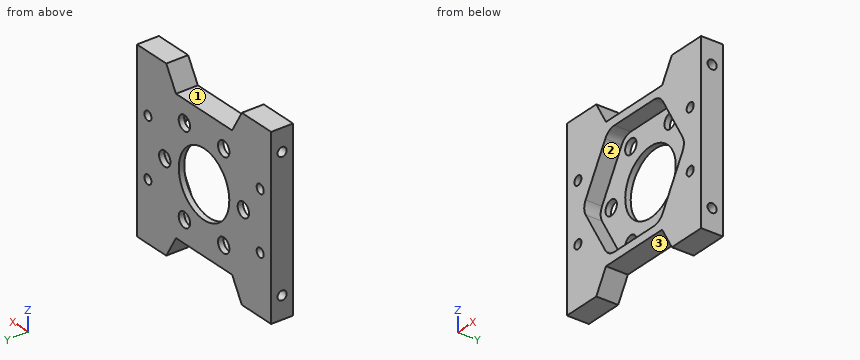
```python
from build123d import *

# Parameters (mm, degrees)
SKETCH_1_R          = 35
SKETCH_1_R_2        = 2.025
SKETCH_1_R_3        = 9
SKETCH_1_R_4        = 1.25
EXTRUDE_1_DEPTH     = 3
CUT_EXTRUDE_1_REACH = 51.86
SKETCH_2_R          = 35
SKETCH_2_W          = 47.8
SKETCH_2_H          = 48.2
SKETCH_3_R          = 1.25
CUT_EXTRUDE_2_DEPTH = 8
SKETCH_5_R          = 9
SKETCH_5_R_2        = 3.75
SKETCH_5_R_3        = 2.025
CUT_EXTRUDE_4_DEPTH = 4.5
CUT_EXTRUDE_6_DEPTH = 35.467666007


with BuildPart() as part:
    # 草图1 → 凸台-拉伸1 (new, symmetric)
    with BuildSketch(Plane(origin=(0, 0, 0), x_dir=(1, 0, 0), z_dir=(0, 1, 0))):
        with Locations(Location((0, 0, 0), (0, 0, 270))):
            Circle(SKETCH_1_R)
        with Locations(Location((14, 0, 0), (0, 0, 270))):
            Circle(SKETCH_1_R_2, mode=Mode.SUBTRACT)
        with Locations(Location((7, -12.124355653, 0), (0, 0, 270))):
            Circle(SKETCH_1_R_2, mode=Mode.SUBTRACT)
        with Locations(Location((-7, -12.124355653, 0), (0, 0, 270))):
            Circle(SKETCH_1_R_2, mode=Mode.SUBTRACT)
        with Locations(Location((-14, 0, 0), (0, 0, 270))):
            Circle(SKETCH_1_R_2, mode=Mode.SUBTRACT)
        with Locations(Location((-7, 12.124355653, 0), (0, 0, 270))):
            Circle(SKETCH_1_R_2, mode=Mode.SUBTRACT)
        with Locations(Location((7, 12.124355653, 0), (0, 0, 270))):
            Circle(SKETCH_1_R_2, mode=Mode.SUBTRACT)
        with Locations(Location((0, 0, 0), (0, 0, 270))):
            Circle(SKETCH_1_R_3, mode=Mode.SUBTRACT)
        with Locations(Location((-20, 8, 0), (0, 0, 270))):
            Circle(SKETCH_1_R_4, mode=Mode.SUBTRACT)
        with Locations(Location((-20, -8, 0), (0, 0, 90))):
            Circle(SKETCH_1_R_4, mode=Mode.SUBTRACT)
        with Locations(Location((20, -8, 0), (0, 0, 270))):
            Circle(SKETCH_1_R_4, mode=Mode.SUBTRACT)
        with Locations(Location((20, 8, 0), (0, 0, 90))):
            Circle(SKETCH_1_R_4, mode=Mode.SUBTRACT)
    extrude(amount=EXTRUDE_1_DEPTH, both=True)

    # 草图2 → 切除-拉伸1 (cut, up to next)
    with BuildSketch(Plane(origin=(0, 3, 0), x_dir=(1, 0, 0), z_dir=(0, 1, 0)), mode=Mode.PRIVATE) as cut_extrude_1_sk1:
        Circle(SKETCH_2_R)
        Rectangle(SKETCH_2_W, SKETCH_2_H, mode=Mode.SUBTRACT)
    cut_extrude_1_tool1 = extrude(cut_extrude_1_sk1.sketch, amount=-CUT_EXTRUDE_1_REACH, mode=Mode.PRIVATE) & part.part
    add(cut_extrude_1_tool1.solids().sort_by_distance((-34.010051, 3, 0))[0], mode=Mode.SUBTRACT)

    # 草图3 → 切除-拉伸2 (cut)
    with BuildSketch(Plane.ZY.offset(23.9)):
        with Locations((18, 0)):
            Circle(SKETCH_3_R)
        with Locations(Location((-18, 0, 0), (0, 0, 180))):
            Circle(SKETCH_3_R)
    cut_extrude_2 = extrude(amount=-CUT_EXTRUDE_2_DEPTH, mode=Mode.SUBTRACT)

    # 草图5 → 切除-拉伸4 (cut)
    # profile 1 of 7: a face of its own
    with BuildSketch(Plane.XZ.offset(3)):
        with BuildLine():
            Line((7, 15.874355653), (-7, 15.874355653))
            ThreePointArc((-7, 15.874355653), (-4.348349571, 14.776006082), (-3.25, 12.124355653))
            ThreePointArc((-3.25, 12.124355653), (-7.970571419, 8.502133804), (-10.247595264, 13.999355653))
            Line((-10.247595264, 13.999355653), (-17.247595264, 1.875))
            ThreePointArc((-17.247595264, 1.875), (-13.029428581, 3.622221849), (-10.25, 0))
            ThreePointArc((-10.25, 0), (-13.029428581, -3.622221849), (-17.247595264, -1.875))
            Line((-17.247595264, -1.875), (-10.247595264, -13.999355653))
            ThreePointArc((-10.247595264, -13.999355653), (-7.970571419, -8.502133804), (-3.25, -12.124355653))
            ThreePointArc((-3.25, -12.124355653), (-4.348349571, -14.776006082), (-7, -15.874355653))
            Line((-7, -15.874355653), (7, -15.874355653))
            ThreePointArc((7, -15.874355653), (4.348349571, -9.472705224), (10.75, -12.124355653))
            ThreePointArc((10.75, -12.124355653), (10.622221849, -13.094927072), (10.247595264, -13.999355653))
            Line((10.247595264, -13.999355653), (17.247595264, -1.875))
            ThreePointArc((17.247595264, -1.875), (10.25, 0), (17.247595264, 1.875))
            Line((17.247595264, 1.875), (10.247595264, 13.999355653))
            ThreePointArc((10.247595264, 13.999355653), (10.622221849, 13.094927072), (10.75, 12.124355653))
            ThreePointArc((10.75, 12.124355653), (4.348349571, 9.472705224), (7, 15.874355653))
        make_face()
        with Locations(Location((0, 0, 0), (0, 0, 270))):
            Circle(SKETCH_5_R, mode=Mode.SUBTRACT)
    # profile 2 of 7: a face of its own
    with BuildSketch(Plane.XZ.offset(3)):
        with Locations((-14, 0)):
            Circle(SKETCH_5_R_2)
        with Locations(Location((-14, 0, 0), (0, 0, 270))):
            Circle(SKETCH_5_R_3, mode=Mode.SUBTRACT)
    # profile 3 of 7: a face of its own
    with BuildSketch(Plane.XZ.offset(3)):
        with Locations((-7, 12.124355653)):
            Circle(SKETCH_5_R_2)
        with Locations(Location((-7, 12.124355653, 0), (0, 0, 270))):
            Circle(SKETCH_5_R_3, mode=Mode.SUBTRACT)
    # profile 4 of 7: a face of its own
    with BuildSketch(Plane.XZ.offset(3)):
        with Locations((7, 12.124355653)):
            Circle(SKETCH_5_R_2)
        with Locations(Location((7, 12.124355653, 0), (0, 0, 270))):
            Circle(SKETCH_5_R_3, mode=Mode.SUBTRACT)
    # profile 5 of 7: a face of its own
    with BuildSketch(Plane.XZ.offset(3)):
        with Locations((14, 0)):
            Circle(SKETCH_5_R_2)
        with Locations(Location((14, 0, 0), (0, 0, 270))):
            Circle(SKETCH_5_R_3, mode=Mode.SUBTRACT)
    # profile 6 of 7: a face of its own
    with BuildSketch(Plane.XZ.offset(3)):
        with Locations((7, -12.124355653)):
            Circle(SKETCH_5_R_2)
        with Locations(Location((7, -12.124355653, 0), (0, 0, 270))):
            Circle(SKETCH_5_R_3, mode=Mode.SUBTRACT)
    # profile 7 of 7: a face of its own
    with BuildSketch(Plane.XZ.offset(3)):
        with Locations((-7, -12.124355653)):
            Circle(SKETCH_5_R_2)
        with Locations(Location((-7, -12.124355653, 0), (0, 0, 270))):
            Circle(SKETCH_5_R_3, mode=Mode.SUBTRACT)
    extrude(amount=-CUT_EXTRUDE_4_DEPTH, mode=Mode.SUBTRACT)

    # 镜向1: 切除-拉伸2 across plane
    add(cut_extrude_2.mirror(Plane(origin=(0, 0, 0), x_dir=(0, 0, 1), z_dir=(1, 0, 0))), mode=Mode.SUBTRACT)

    # 草图7 → 切除-拉伸6 (cut, through all)
    with BuildSketch(Plane.XZ.offset(3)):
        Polygon((-13.464101615, 24.1), (-10, 18.1), (10, 18.1), (13.464101615, 24.1), align=None)
        Polygon((10, -18.1), (-10, -18.1), (-13.464101615, -24.1), (13.464101615, -24.1), align=None)
    extrude(amount=-CUT_EXTRUDE_6_DEPTH, mode=Mode.SUBTRACT)


solid = part.part
```
Here's how the part is built. I have some questions about the finished solid (model axes, mm). Face numbers are marked on the shaded views. A direction names the side the tool comes from. Give positions to 0.01 mm unless a question says otherwise; leave off trailing zeros. Loops run counter-clockwise (first coordinate to the right, second up) from the corner with the lowest first, then second, coordinate; pieces in that order, holes last. Notation, with made-up numbers: M 41,39.5 L 78,39.5 A23 cw 78,58.5 Z; hole C 5,73.25 d10. An arc over 180 degrees is marked long. Use one line per item in the form item = value. Start each with the question number.
Q1. If we section it at D-D (x = 15): Write out the boundary of the cut face in (y, z).
Q2. If we section it at A-A (x = 20): Write out the boundary of the cut face in (y, z), then the cut area to 3 significant figures.
Q3. If we section it at C-C (y = -2): Write out the boundary of the cut face in (x, z) (3 decimals), then the cut area to 3 significant figures.
Q4. I need wall thicknesses on line 1 along X through (y, z) = (2.4, 0) (3 decimals); line 2 along X through (y, z) = (1.2, -21.5); line 3 along Z through (x, y) = (-7, -2.3). Which ranges of each line are inside material? Lowest first, please.
Q5. Which directions (+Z, -Z, +X, -X, +Y, -Y) give clear straight access to the entire face, cutting with the end or side of a thin tool? Please do the marked faces 1, 2 and 3.
Q6. If we section it at B-B (z = 0): Write out the boundary of the cut face in (x, y) (3 decimals), then the cut area to 3 significant figures.
Q7. Will these pins go through, and if not, where does the flat tip stop? pin 1 Ø2.5 at (x, z) = (-14, 0) entering from +Y; pin 2 Ø3 at (x, y) = (5, -1.5) entering from +Z; pin 3 Ø3 at (x, y) = (-3, 1.5) entering from -Z.
Taken from the geometry:
q1.outline = M -3,-24.1 L 3,-24.1 L 3,-1.76 L 1.5,-1.76 L 1.5,-5.77 L -3,-5.77 Z; M -3,5.77 L 1.5,5.77 L 1.5,1.76 L 3,1.76 L 3,24.1 L -3,24.1 Z
q2.outline = M -3,-24.1 L 3,-24.1 L 3,-9.25 L -3,-9.25 Z; M -3,-6.75 L 3,-6.75 L 3,6.75 L -3,6.75 Z; M -3,9.25 L 3,9.25 L 3,24.1 L -3,24.1 Z; hole C 0,-18 d2.5; hole C 0,18 d2.5
q2.area = 249 mm^2
q3.outline = M -23.9,-24.1 L -13.464,-24.1 L -10,-18.1 L 10,-18.1 L 13.464,-24.1 L 23.9,-24.1 L 23.9,24.1 L 13.464,24.1 L 10,18.1 L -10,18.1 L -13.464,24.1 L -23.9,24.1 Z; hole C -20,-8 d2.5; hole C -20,8 d2.5; hole M -17.248,-1.875 L -10.248,-13.999 A3.75 ccw -7,-15.874 L 7,-15.874 A3.75 ccw 10.248,-13.999 L 17.248,-1.875 A3.75 ccw 17.248,1.875 L 10.248,13.999 A3.75 ccw 7,15.874 L -7,15.874 A3.75 ccw -10.248,13.999 L -17.248,1.875 A3.75 ccw Z; hole C 20,-8 d2.5; hole C 20,8 d2.5
q3.area = 1,130 mm^2
q4.line_1 = -23.9 to -16.025, -11.975 to -9, 9 to 11.975, 16.025 to 23.9
q4.line_2 = -23.9 to -11.96, 11.96 to 23.9
q4.line_3 = -18.1 to -15.87, 15.87 to 18.1
q5.face_1 = +Z, +Y, -Y
q5.face_2 = -Y
q5.face_3 = -Z, +Y, -Y
q6.outline = M -23.9,-3 L -17.75,-3 L -17.75,1.5 L -16.025,1.5 L -16.025,3 L -23.9,3 Z; M -11.975,1.5 L -9,1.5 L -9,3 L -11.975,3 Z; M 9,1.5 L 11.975,1.5 L 11.975,3 L 9,3 Z; M 16.025,1.5 L 17.75,1.5 L 17.75,-3 L 23.9,-3 L 23.9,3 L 16.025,3 Z
q6.area = 87.9 mm^2
q7.pin_1 = through
q7.pin_2 = 18.1
q7.pin_3 = -18.1
